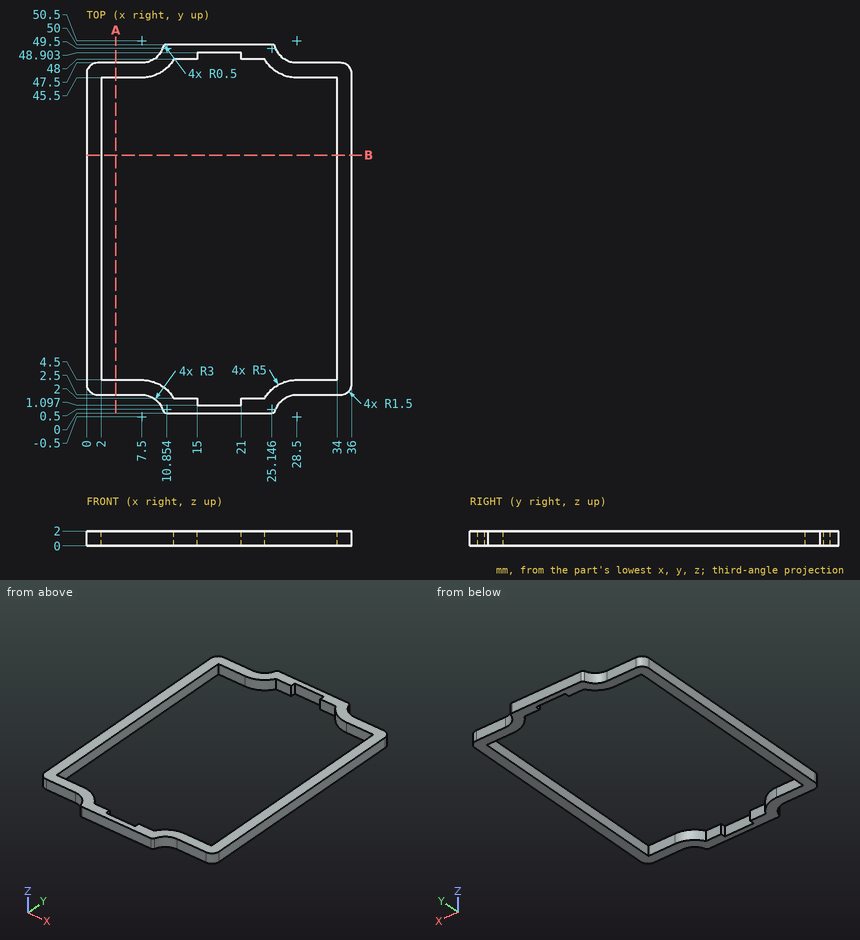
Drawing for the job (mm, zero at the part's lowest x, y, z). Give positions to 0.01 mm unless a question says otherwise; leave off trailing zeros. Order: outer loops, then holes, each group sorted by start corner. A loop starts at its lowest first (then second) coordinate and runs counter-clockwise, first axis right, second up. Notation, with made-up numbers: M 31.25,62.25 L 45.25,62.25 A27 cw 45.25,79.25 Z; hole C 10,-3.75 d7. An arc over 180 degrees is marked long. Use a Markdown table: item, result. Add a question column.
(1) Probe line 1 along X through (y, z) = (32, 0.55); line 2 along Y through (x, z) = (17.5, 0.85); line 3 along Y through (x, z) = (21.5, 1.9). List the from-to ranges inside material, lowest first. Write a range as [from, to].
(2) Drop flat-ended pins along their axis: P1, Ø0.6, axis at x = 4, z = 0.5, coming from the +Y side; P2, Ø0.5, axis at y = 1.5, z = 1.5, coming from the -X side; P3, Ø10, axis at x = 12.5, y = 38.5, coming from the +Z side; P4, Ø1, axis at x = 6, z = 1, coming from the -Y side. Give the stop position or say it passes through.
(3) Saw through at B-B, the plane y = 35. Give the cut face in (x, z).
(4) Saw through at A-A, the plane x = 4. Give the cut face in (y, z).
Answer key:
| question | item | result |
|---|---|---|
| 1 | line 1 | [0, 2], [34, 36] |
| 1 | line 2 | [0, 1.1], [48.9, 50] |
| 1 | line 3 | [0, 2], [48, 50] |
| 2 | P1 | y = 47.5 |
| 2 | P2 | x = 9.48 |
| 2 | P3 | through |
| 2 | P4 | y = 2.5 |
| 3 | outline | M 0,0 L 2,0 L 2,2 L 0,2 Z; M 34,0 L 36,0 L 36,2 L 34,2 Z |
| 4 | outline | M 2.5,0 L 4.5,0 L 4.5,2 L 2.5,2 Z; M 45.5,0 L 47.5,0 L 47.5,2 L 45.5,2 Z |
